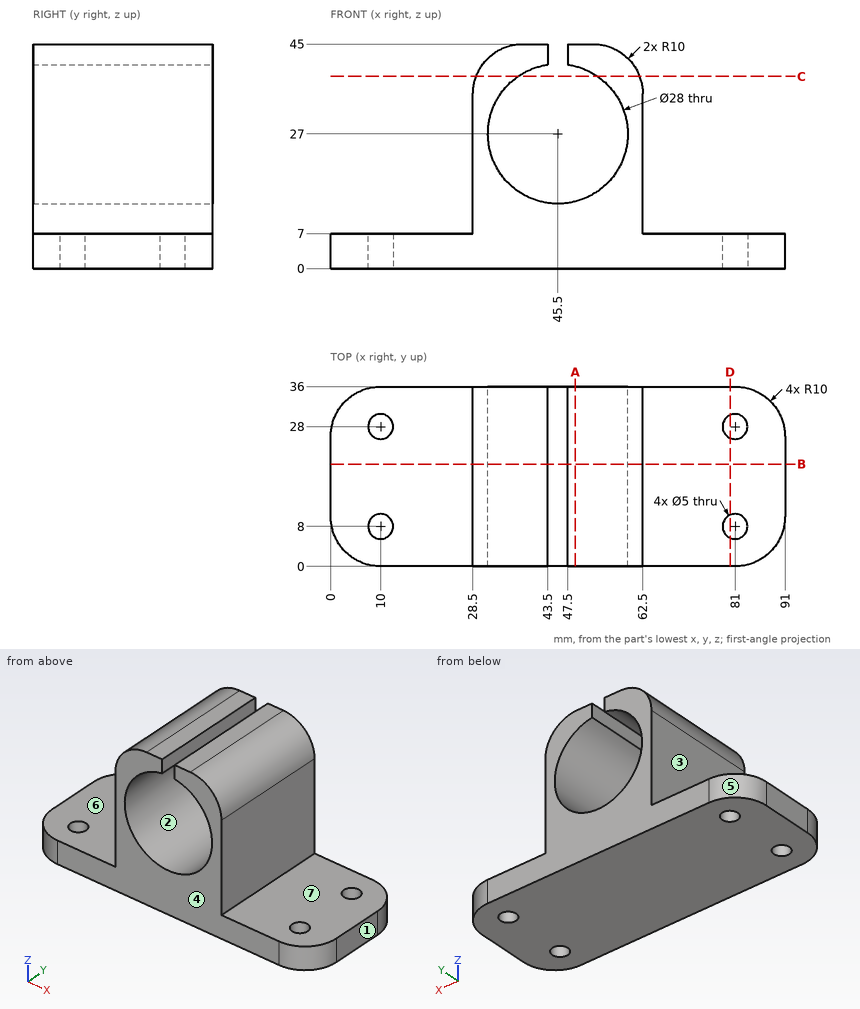
Here's the drawing with two shaded views (mm, measured from the low corner). I have some questions. A direction names the side the tool comes from. Coordinates: 2 decimals unless noted, no trailing zeros. Write each loop counter-clockwise with the first axis right and the second up, starting at its lowest first coordinate (ties: lowest second). Pieces come first, ordered by that corner, then holes. Notation, with made-up numbers: (48, 21.25) - (53, 21.25) arc R21 ccw to (53, 49.25) - close; hole circle Ø10 at (-24, 4). An arc over 180 degrees is marked (long way). Return JSON: item names as keys, results as strings.
Q1. If we section it at C-C (z = 38.5): Please give me the cut outline in (x, y), then the cut area to 3 significant figures.
Computed values:
{"outline": "(29.13, 0) - (37.52, 0) - (37.52, 36) - (29.13, 36) - close; (53.48, 0) - (61.87, 0) - (61.87, 36) - (53.48, 36) - close", "area": "604 mm2"}
Q2. Thinking about a two-plate mould opening in X: for the marked faces 1, 2, 3 and 4, which applies, +X half, -X half, draft (parallel to the pull), parting line (faces both ways), or undercut?
Computed values:
{"face 1": "+X half", "face 2": "undercut", "face 3": "-X half", "face 4": "draft"}
Q3. Please list where these lines run through material, in increasing order: L1, parallel to Y at x = 81, z = 2; L2, parallel to X at y = 28, z = 27; L3, parallel to Z at x = 17, y = 21. Write a range as from..to.
Computed values:
{"L1": "y = 0..5.5, 10.5..25.5, 30.5..36", "L2": "x = 28.5..31.5, 59.5..62.5", "L3": "z = 0..7"}
Q4. If we section it at A-A (x = 49): Please give me the cut outline in (y, z).
Computed values:
{"outline": "(0, 0) - (36, 0) - (36, 13.44) - (0, 13.44) - close; (0, 40.56) - (36, 40.56) - (36, 45) - (0, 45) - close"}
Q5. On a 3-axis mill with a long thin cutter (end or side, diameter ignored), from which of +Z, -Z, +X, -X, +Y, -Y can I reach the whole of each face in a straight line? I mean the marked faces 5, 6 and 7. Say none if no direction works.
Computed values:
{"face 5": "+Z, -Z, -X, +Y", "face 6": "+Z, -X, +Y, -Y", "face 7": "+Z, +X, +Y, -Y"}
Q6. I'm going to push flat-ended pins straight in: pin 1 Ø2 at (y, z) = (5.5, 27.5) entering from -X; pin 2 Ø14 at (y, z) = (20, 26) entering from +X; pin 3 Ø8.5 at (x, y) = (76, 9.5) entering from +Z. Where does each tip first touch, or does it pass through?
Computed values:
{"pin 1": "stops at x = 28.5", "pin 2": "stops at x = 62.5", "pin 3": "stops at z = 7"}
Q7. If we section it at D-D (x = 80): Please give me the cut outline in (y, z), then the cut area to 3 significant figures.
Computed values:
{"outline": "(0, 0) - (5.71, 0) - (5.71, 7) - (0, 7) - close; (10.29, 0) - (25.71, 0) - (25.71, 7) - (10.29, 7) - close; (30.29, 0) - (36, 0) - (36, 7) - (30.29, 7) - close", "area": "188 mm2"}
Q8. If we section it at B-B (y = 20.5): Please give me the cut outline in (x, z).
Computed values:
{"outline": "(0, 0) - (91, 0) - (91, 7) - (62.5, 7) - (62.5, 35) arc R10 ccw to (52.5, 45) - (47.5, 45) - (47.5, 40.86) arc R14 cw (long way) to (43.5, 40.86) - (43.5, 45) - (38.5, 45) arc R10 ccw to (28.5, 35) - (28.5, 7) - (0, 7) - close"}
